from build123d import *

# Parameters (mm, degrees)
CROQUIS1_W                       = 46.3
CROQUIS1_H                       = 42.3
CROQUIS1_R                       = 11.5
CROQUIS1_R_2                     = 1.25
BRIDA_BASE1_DEPTH                = 3
STRUCTURE_SUPORT_STRIP_W         = 14
STRUCTURE_SUPORT_STRIP_H         = 3
STRUCTURE_SUPORT_STRIP_CUT_DEPTH = 42.3
STRUCTURE_SUPORT_DEPTH           = 42.3
STRUCTURE_SUPORT_FLAT_DEPTH      = 3
CROQUIS13_R                      = 1.75
CORTAR_EXTRUIR2_DEPTH            = 57.94168596
DESDOBLAR2_DEPTH                 = 17
DESDOBLAR2_START                 = -3
DESDOBLAR2_2_DEPTH               = 3
DOBLAR2_START                    = -41.076990817
DOBLAR2_OUTLINE_W                = 57.8
DOBLAR2_OUTLINE_H                = 3
DOBLAR2_DEPTH                    = 16
DOBLAR2_START_2                  = -24.77248
DOBLAR2_2_DEPTH                  = 2.62248
DOBLAR2_START_3                  = -25.15
DOBLAR2_3_DEPTH                  = 4
DOBLAR2_START_4                  = -34
DOBLAR2_4_DEPTH                  = 68
CHAFL_N1_SIZE                    = 4
TALADRO_DE_MARGEN_PARA_M31_D     = 3.2
CORTAR_EXTRUIR6_REACH            = 58.942
REDONDEO2_R                      = 0.5


with BuildPart() as part:
    # Brida base1: sheet metal written as solids
    # Croquis1 → Brida base1 (new body)
    with BuildSketch(Plane.XY):
        with Locations((-2, 0)):
            Rectangle(CROQUIS1_W, CROQUIS1_H)
        Circle(CROQUIS1_R, mode=Mode.SUBTRACT)
        with Locations((-15.5, 15.5)):
            Circle(CROQUIS1_R_2, mode=Mode.SUBTRACT)
        with Locations((-15.5, -15.5)):
            Circle(CROQUIS1_R_2, mode=Mode.SUBTRACT)
        with Locations((15.5, -15.5)):
            Circle(CROQUIS1_R_2, mode=Mode.SUBTRACT)
        with Locations((15.5, 15.5)):
            Circle(CROQUIS1_R_2, mode=Mode.SUBTRACT)
    extrude(amount=-BRIDA_BASE1_DEPTH)

    # Structure Suport: sheet metal written as solids
    # Structure Suport strip (on a plane across the edge) → Structure Suport strip cut (cut)
    with BuildSketch(Plane(origin=(-25.15, 21.15, 0), x_dir=(1, 0, 0), z_dir=(0, -1, 0))):
        with Locations((-3, -1.5)):
            Rectangle(STRUCTURE_SUPORT_STRIP_W, STRUCTURE_SUPORT_STRIP_H)
    extrude(amount=STRUCTURE_SUPORT_STRIP_CUT_DEPTH, mode=Mode.SUBTRACT)

    # Structure Suport bend section (on a plane across the edge) → Structure Suport (add)
    with BuildSketch(Plane(origin=(-25.15, 21.15, 0), x_dir=(1, 0, 0), z_dir=(0, -1, 0))):
        with BuildLine():
            Line((0, 1), (3, 1))
            ThreePointArc((3, 1), (3.292893219, 0.292893219), (4, 0))
            Line((4, 0), (4, -3))
            ThreePointArc((4, -3), (1.171572875, -1.828427125), (0, 1))
        make_face()
    extrude(amount=STRUCTURE_SUPORT_DEPTH)

    # Structure Suport profile (on flange) → Structure Suport flat (add)
    with BuildSketch(Plane(origin=(-25.15, 0, 0), x_dir=(0, -1, 0), z_dir=(-1, 0, 0))):
        with BuildLine():
            ThreePointArc((-26.34, 17), (-32.84, 10.5), (-26.34, 4))
            Line((-26.34, 4), (-21.15, 4))
            Line((-21.15, 4), (-21.15, 1))
            Line((-21.15, 1), (21.15, 1))
            Line((21.15, 1), (21.15, 4))
            Line((21.15, 4), (26.34, 4))
            ThreePointArc((26.34, 4), (32.84, 10.5), (26.34, 17))
            Line((26.34, 17), (-26.34, 17))
        make_face()
    extrude(amount=-STRUCTURE_SUPORT_FLAT_DEPTH)

    # Croquis13 → Cortar-Extruir2 (cut, through all)
    with BuildSketch(Plane(origin=(-22.15, 0, 0), x_dir=(0, 0, -1), z_dir=(1, 0, 0))):
        with Locations((-10.5, 27.15)):
            Circle(CROQUIS13_R)
        with BuildLine():
            Line((-10.5, 28.9), (-12.25, 28.9))
            ThreePointArc((-12.25, 28.9), (-14, 27.15), (-12.25, 25.4))
            Line((-12.25, 25.4), (-10.5, 25.4))
            ThreePointArc((-10.5, 25.4), (-12.25, 27.15), (-10.5, 28.9))
        make_face()
        with BuildLine():
            Line((-8.75, 28.9), (-10.5, 28.9))
            ThreePointArc((-10.5, 28.9), (-9.262563133, 28.387436867), (-8.75, 27.15))
            ThreePointArc((-8.75, 27.15), (-9.262563133, 25.912563133), (-10.5, 25.4))
            Line((-10.5, 25.4), (-8.75, 25.4))
            ThreePointArc((-8.75, 25.4), (-7, 27.15), (-8.75, 28.9))
        make_face()
        with Locations((-10.5, -27.15)):
            Circle(CROQUIS13_R)
        with BuildLine():
            Line((-10.5, -25.4), (-12.25, -25.4))
            ThreePointArc((-12.25, -25.4), (-14, -27.15), (-12.25, -28.9))
            Line((-12.25, -28.9), (-10.5, -28.9))
            ThreePointArc((-10.5, -28.9), (-12.25, -27.15), (-10.5, -25.4))
        make_face()
        with BuildLine():
            Line((-8.75, -25.4), (-10.5, -25.4))
            ThreePointArc((-10.5, -25.4), (-9.262563133, -25.912563133), (-8.75, -27.15))
            ThreePointArc((-8.75, -27.15), (-9.262563133, -28.387436867), (-10.5, -28.9))
            Line((-10.5, -28.9), (-8.75, -28.9))
            ThreePointArc((-8.75, -28.9), (-7, -27.15), (-8.75, -25.4))
        make_face()
    extrude(amount=-CORTAR_EXTRUIR2_DEPTH, mode=Mode.SUBTRACT)

    # Desdoblar2: read off the stored shape, not the designer's step
    # Desdoblar2 outline → Desdoblar2 (cut)
    with BuildSketch(Plane.XY):
        Polygon((-25.15, -34), (-22.15, -34), (-22.15, -21.15), (-20, -21.15), (-20, 21.15), (-22.15, 21.15), (-22.15, 34), (-25.15, 34), align=None)
    extrude(amount=DESDOBLAR2_DEPTH, mode=Mode.SUBTRACT)

    # Desdoblar2 2 outline → Desdoblar2 2 (add)
    with BuildSketch(Plane.XY.offset(DESDOBLAR2_START)):
        with BuildLine():
            Line((-28.076990817, 21.15), (-28.076990817, 26.34))
            ThreePointArc((-28.076990817, 26.34), (-34.576990817, 32.84), (-41.076990817, 26.34))
            Line((-41.076990817, 26.34), (-41.076990817, -26.34))
            ThreePointArc((-41.076990817, -26.34), (-34.576990817, -32.84), (-28.076990817, -26.34))
            Line((-28.076990817, -26.34), (-28.076990817, -21.15))
            Line((-28.076990817, -21.15), (-20, -21.15))
            Line((-20, -21.15), (-20, 21.15))
            Line((-20, 21.15), (-28.076990817, 21.15))
        make_face()
        with BuildLine():
            Line((-36.326990817, -25.4), (-32.826990817, -25.4))
            ThreePointArc((-32.826990817, -25.4), (-31.076990817, -27.15), (-32.826990817, -28.9))
            Line((-32.826990817, -28.9), (-36.326990817, -28.9))
            ThreePointArc((-36.326990817, -28.9), (-38.076990817, -27.15), (-36.326990817, -25.4))
        make_face(mode=Mode.SUBTRACT)
        with BuildLine():
            Line((-32.826990817, 25.4), (-36.326990817, 25.4))
            ThreePointArc((-36.326990817, 25.4), (-38.076990817, 27.15), (-36.326990817, 28.9))
            Line((-36.326990817, 28.9), (-32.826990817, 28.9))
            ThreePointArc((-32.826990817, 28.9), (-31.076990817, 27.15), (-32.826990817, 25.4))
        make_face(mode=Mode.SUBTRACT)
    extrude(amount=DESDOBLAR2_2_DEPTH)

    # Doblar2: read off the stored shape, not the designer's step
    # Doblar2 outline → Doblar2 (cut)
    with BuildSketch(Plane.YZ.offset(DOBLAR2_START)):
        with Locations((0, -1.5)):
            Rectangle(DOBLAR2_OUTLINE_W, DOBLAR2_OUTLINE_H)
    extrude(amount=DOBLAR2_DEPTH, mode=Mode.SUBTRACT)

    # Doblar2 2 outline → Doblar2 2 (add)
    with BuildSketch(Plane.YZ.offset(DOBLAR2_START_2)):
        with BuildLine():
            Line((21.15, 0), (21.15, 4))
            Line((21.15, 4), (26.34, 4))
            ThreePointArc((26.34, 4), (32.84, 10.5), (26.34, 17))
            Line((26.34, 17), (-26.34, 17))
            ThreePointArc((-26.34, 17), (-32.84, 10.5), (-26.34, 4))
            Line((-26.34, 4), (-21.15, 4))
            Line((-21.15, 4), (-21.15, 0))
            Line((-21.15, 0), (21.15, 0))
        make_face()
        with BuildLine():
            ThreePointArc((-28.9, 12.25), (-27.15, 14), (-25.4, 12.25))
            Line((-25.4, 12.25), (-25.4, 8.75))
            ThreePointArc((-25.4, 8.75), (-27.15, 7), (-28.9, 8.75))
            Line((-28.9, 8.75), (-28.9, 12.25))
        make_face(mode=Mode.SUBTRACT)
        with BuildLine():
            ThreePointArc((25.4, 12.25), (27.15, 14), (28.9, 12.25))
            Line((28.9, 12.25), (28.9, 8.75))
            ThreePointArc((28.9, 8.75), (27.15, 7), (25.4, 8.75))
            Line((25.4, 8.75), (25.4, 12.25))
        make_face(mode=Mode.SUBTRACT)
    extrude(amount=DOBLAR2_2_DEPTH)

    # Doblar2 3 outline → Doblar2 3 (add)
    with BuildSketch(Plane.YZ.offset(DOBLAR2_START_3)):
        with BuildLine():
            Line((21.15, 0), (21.15, 4))
            Line((21.15, 4), (26.34, 4))
            ThreePointArc((26.34, 4), (32.84, 10.5), (26.34, 17))
            Line((26.34, 17), (-26.34, 17))
            ThreePointArc((-26.34, 17), (-32.84, 10.5), (-26.34, 4))
            Line((-26.34, 4), (-21.15, 4))
            Line((-21.15, 4), (-21.15, 0))
            Line((-21.15, 0), (21.15, 0))
        make_face()
        with BuildLine():
            ThreePointArc((-28.9, 12.25), (-27.15, 14), (-25.4, 12.25))
            Line((-25.4, 12.25), (-25.4, 8.75))
            ThreePointArc((-25.4, 8.75), (-27.15, 7), (-28.9, 8.75))
            Line((-28.9, 8.75), (-28.9, 12.25))
        make_face(mode=Mode.SUBTRACT)
        with BuildLine():
            ThreePointArc((25.4, 12.25), (27.15, 14), (28.9, 12.25))
            Line((28.9, 12.25), (28.9, 8.75))
            ThreePointArc((28.9, 8.75), (27.15, 7), (25.4, 8.75))
            Line((25.4, 8.75), (25.4, 12.25))
        make_face(mode=Mode.SUBTRACT)
    extrude(amount=DOBLAR2_3_DEPTH)

    # Doblar2 4 outline → Doblar2 4 (cut)
    with BuildSketch(Plane(origin=(0, 0, 0), x_dir=(1, 0, 0), z_dir=(0, 1, 0)).offset(DOBLAR2_START_4)):
        with BuildLine():
            ThreePointArc((-21.15, 0), (-21.857106781, -0.292893219), (-22.15, -1))
            Line((-22.15, -1), (-22.15, -17))
            Line((-22.15, -17), (-21.15, -17))
            Line((-21.15, -17), (-21.15, 0))
        make_face()
        with BuildLine():
            Line((-25.15, -17), (-25.15, -1))
            ThreePointArc((-25.15, -1), (-23.978427125, 1.828427125), (-21.15, 3))
            Line((-21.15, 3), (-20, 3))
            Line((-20, 3), (-20, 5))
            Line((-20, 5), (-42, 5))
            Line((-42, 5), (-42, -17))
            Line((-42, -17), (-25.15, -17))
        make_face()
    extrude(amount=DOBLAR2_4_DEPTH, mode=Mode.SUBTRACT)

    # Chaflán1
    chafl_n1_edges = [part.edges().sort_by_distance(p)[0] for p in [
        (21.15, 21.15, -1.5),
        (21.15, -21.15, -1.5),
    ]]
    chamfer(chafl_n1_edges, length=CHAFL_N1_SIZE)

    # Taladro de margen para M31 (through all)
    with Locations(Plane(origin=(0, 0, -3), x_dir=(-1, 0, 0), z_dir=(0, 0, -1))):
        with Locations((9.899494937, -9.899494937), (-9.899494937, -9.899494937), (-9.899494937, 9.899494937), (9.899494937, 9.899494937)):
            Hole(TALADRO_DE_MARGEN_PARA_M31_D / 2)

    # Croquis34 → Cortar-Extruir6 (cut, up to next)
    with BuildSketch(Plane(origin=(-22.15, 0, 0), x_dir=(0, 0, -1), z_dir=(1, 0, 0)), mode=Mode.PRIVATE) as cortar_extruir6_sk1:
        with BuildLine():
            Line((-6, 21.15), (-4, 21.15))
            Line((-4, 21.15), (-4, 22.15))
            Line((-4, 22.15), (-6, 22.15))
            ThreePointArc((-6, 22.15), (-6.5, 21.65), (-6, 21.15))
        make_face()
    cortar_extruir6_tool1 = extrude(cortar_extruir6_sk1.sketch, amount=-CORTAR_EXTRUIR6_REACH, mode=Mode.PRIVATE) & part.part
    # Croquis34 → Cortar-Extruir6 (cut, up to next)
    with BuildSketch(Plane(origin=(-22.15, 0, 0), x_dir=(0, 0, -1), z_dir=(1, 0, 0)), mode=Mode.PRIVATE) as cortar_extruir6_sk2:
        with BuildLine():
            Line((-4, -22.15), (-6, -22.15))
            ThreePointArc((-6, -22.15), (-6.5, -21.65), (-6, -21.15))
            Line((-6, -21.15), (-4, -21.15))
            Line((-4, -21.15), (-4, -22.15))
        make_face()
    cortar_extruir6_tool2 = extrude(cortar_extruir6_sk2.sketch, amount=-CORTAR_EXTRUIR6_REACH, mode=Mode.PRIVATE) & part.part
    add(cortar_extruir6_tool1.solids().sort_by_distance((-22.15, 21.65, 5.198952))[0], mode=Mode.SUBTRACT)
    add(cortar_extruir6_tool2.solids().sort_by_distance((-22.15, -21.65, 5.198952))[0], mode=Mode.SUBTRACT)

    # Redondeo2
    redondeo2_edges = [part.edges().sort_by_distance(p)[0] for p in [
        (21.15, -17.15, -1.5),
        (21.15, 17.15, -1.5),
        (17.15, 21.15, -1.5),
        (17.15, -21.15, -1.5),
        (-23.65, -22.15, 4),
        (-23.65, 22.15, 4),
    ]]
    fillet(redondeo2_edges, radius=REDONDEO2_R)


solid = part.part
Design review of the part built by this model. Coordinates are the model's own, in mm. A direction names the side the tool comes from. Coordinates: 2 decimals unless noted, no trailing zeros. Loops run counter-clockwise (first coordinate to the right, second up) from the corner with the lowest first, then second, coordinate; pieces in that order, holes last.
Item 1: Add section B-B (x = -15.5). Write out the cut boundary in (y, z).
Completed:
outline: (-21.15, -3) - (-16.75, -3) - (-16.75, 0) - (-21.15, 0) - close; (-14.25, -3) - (14.25, -3) - (14.25, 0) - (-14.25, 0) - close; (16.75, -3) - (21.15, -3) - (21.15, 0) - (16.75, 0) - close
Item 2: Add section A-A (y = -15.5). Write out the cut boundary in (x, z), and give its area (3 significant figures).
Completed:
outline: (-25.15, 1) arc R4 ccw to (-21.15, -3) - (-16.75, -3) - (-16.75, 0) - (-21.15, 0) arc R1 cw to (-22.15, 1) - (-22.15, 17) - (-25.15, 17) - close; (-14.25, -3) - (14.25, -3) - (14.25, 0) - (-14.25, 0) - close; (16.75, -3) - (21.15, -3) - (21.15, 0) - (16.75, 0) - close
area: 172 mm2
Item 3: Wall thickness on L1, parallel to Y at x = -15.5, z = -0.8; L2, parallel to X at y = 14.5, z = -2; L3, parallel to Z at x = 17, y = -4: over which ranges is each line inside the solid? List them lowest first.
Completed:
L1: y = -21.15 to -16.75, -14.25 to 14.25, 16.75 to 21.15
L2: x = -23.8 to -16.25, -14.75 to 14.75, 16.25 to 21.15
L3: z = -3 to 0
Item 4: Add section C-C (y = 2). Write out the cut boundary in (x, z), and give its area (3 significant figures).
Completed:
outline: (-25.15, 1) arc R4 ccw to (-21.15, -3) - (-11.32, -3) - (-11.32, 0) - (-21.15, 0) arc R1 cw to (-22.15, 1) - (-22.15, 17) - (-25.15, 17) - close; (11.32, -3) - (21.15, -3) - (21.15, 0) - (11.32, 0) - close
area: 119 mm2
Item 5: Clearance check with flat-ended pins moving along their axes: pin 1 (10 mm diameter, centred on x = 1, y = 24.5, fed in from +Z); pin 2 (4.5 mm diameter, centred on x = -9.5, z = 2, fed in from -Y); pin 3 (4 mm diameter, centred on y = 13, z = 14, fed in from +X); pin 4 (12.5 mm diameter, centred on x = 2.5, y = 4, fed in from +Z). State where each tip first meets the part, or that it passes through.
Completed:
pin 1: stops at z = 0
pin 2: stops at y = -21.15
pin 3: stops at x = -22.15
pin 4: passes through
Item 6: For faces 4 (the cylindrical face through (-1.5, 11.4, -1.5)), 5 (the cylindrical face through (-23.7, -27.1, 7)), 6 (the flat face through (-24, -22.15, 5)), list the 3-axis set-ups (+Z, -Z, +X, -X, +Y, -Y) from which the entire face can be reached by the end or side of a thin tool; tool diameter is ignored.
Completed:
face 4: +Z, -Z
face 5: +X, -X
face 6: -Z, +X, -X
Item 7: Draft analysis for pull direction Y (two halves, no side actions). For faces 1 (the cylindrical face through (-23.7, 27.2, 7)), 2 (the flat face through (-24, 24, 4)), 3 (the cylindrical face through (-23.67, 32.84, 10.36)), state which applies: pulls with the +Y half, pulls with the -Y half, needs draft (parallel to the pull), parting line crosses it, or undercut.
Completed:
face 1: undercut
face 2: needs draft
face 3: pulls with the +Y half
Item 8: Add section D-D (x = 1). Write out the cut boundary in (y, z), and give its area (3 significant figures).
Completed:
outline: (-21.15, -3) - (-11.46, -3) - (-11.46, 0) - (-21.15, 0) - close; (11.46, -3) - (21.15, -3) - (21.15, 0) - (11.46, 0) - close
area: 58.2 mm2
